Autodesk Inventor part; units mm, degrees
ref_plane "YZ Plane" through (0, 0, 0) normal (1, 0, 0) x (0, 1, 0)
ref_plane "XZ Plane" through (0, 0, 0) normal (0, 1, 0) x (-1, 0, 0)
ref_plane "XY Plane" through (0, 0, 0) normal (0, 0, 1) x (1, 0, 0)
sketch "Sketch2" plane through (0, 0, 0) normal (0, 0, 1) x (1, 0, 0)
  line L0 (-108, -20.3137) -> (62, -20.3137) construction
  line L1 (-108, -35.3137) -> (62, -35.3137)
  line L2 (62, -5.3137) -> (-108, -5.3137)
  arc A0 (-108, -5.3137) -> (-108, -35.3137) centre (-108, -20.3137) ccw
  arc A1 (62, -35.3137) -> (62, -5.3137) centre (62, -20.3137) ccw
  circle A2 centre (-108, -20.3137) radius 10
  circle A3 centre (62, -20.3137) radius 10
  line L3 (-84, -20.3137) -> (-68, -20.3137) construction
  line L4 (-84, -27.8137) -> (-68, -27.8137)
  line L5 (-68, -12.8137) -> (-84, -12.8137)
  arc A4 (-84, -12.8137) -> (-84, -27.8137) centre (-84, -20.3137) ccw
  arc A5 (-68, -27.8137) -> (-68, -12.8137) centre (-68, -20.3137) ccw
  line L6 (-23, -46) -> (-23, 6) construction
  arc A6 (-33, -27.8137) -> (-33, -12.8137) centre (-33, -20.3137) ccw
  line L7 (-49, -20.3137) -> (-33, -20.3137) construction
  line L8 (-49, -27.8137) -> (-33, -27.8137)
  line L9 (-33, -12.8137) -> (-49, -12.8137)
  arc A7 (-49, -12.8137) -> (-49, -27.8137) centre (-49, -20.3137) ccw
  line L10 (38, -20.3137) -> (22, -20.3137) construction
  line L11 (38, -27.8137) -> (22, -27.8137)
  line L12 (22, -12.8137) -> (38, -12.8137)
  arc A8 (38, -27.8137) -> (38, -12.8137) centre (38, -20.3137) ccw
  arc A9 (22, -12.8137) -> (22, -27.8137) centre (22, -20.3137) ccw
  arc A10 (-13, -12.8137) -> (-13, -27.8137) centre (-13, -20.3137) ccw
  line L13 (3, -20.3137) -> (-13, -20.3137) construction
  line L14 (3, -27.8137) -> (-13, -27.8137)
  line L15 (-13, -12.8137) -> (3, -12.8137)
  arc A11 (3, -27.8137) -> (3, -12.8137) centre (3, -20.3137) ccw
  line L16 (-121.6954, -14.1952) -> (-147.279, -14.1952)
  line L17 (-121.6954, -26.4323) -> (-147.279, -26.4323)
  circle A12 centre (-154, -20.3137) radius 9.0889
  circle A13 centre (-108, -20.3137) radius 12.5
  line L18 (-119.5282, -20.3137) -> (-121.5282, -20.3137)
  point P0 (0, 0)
  point P1 (-23, -20.3137)
  point P2 (-76, -20.3137)
  point P3 (-41, -20.3137)
  point P4 (30, -20.3137)
  point P5 (-5, -20.3137)
  point P6 (-120.5, -20.3137)
  dimension "d51" = 25
  dimension "d27" = 170
  dimension "d28" = 30
  dimension "d29" = 20
  dimension "d30" = 20
  dimension "d31" = 16
  dimension "d32" = 15
  dimension "d43" = 35
  dimension "d48" = 40
  dimension "d57" = 2
extrude "Extrusion2" add sketch "Sketch2" along normal blind 3 contours A0 L2 A1 L1 | L17 A12 L16 A0 | A12 | A13
extrude "Extrusion3" add sketch "Sketch2" against normal blind 3 contours A13
ref_plane "Work Plane1" through (-119.5282, -20.3137, 0) normal (0, -1, 0) x (-1, 0, 0)
sketch "Sketch4" plane through (-108, -20.3137, -3) normal (0, 0, -1) x (-1, 0, 0)
  line L0 (11.5282, 0) -> (13.5282, 0)
  circle A0 centre (0, 0) radius 12.5
  point P0 (-108, 20.3137)
  point P1 (12.5, 0)
ref_plane "Work Plane2" through (-120.5, -20.3137, -3) normal (-1, 0, 0) x (0, -1, 0)
sketch "Sketch5" plane through (-120.5, -20.3137, -3) normal (-1, 0, 0) x (0, -1, 0)
  line L0 (9.0889, 3) -> (-9.0889, 3)
  line L1 (-12.5, 0) -> (12.5, 0)
  line L2 (0, -1.2) -> (0, 7.2)
  line L3 (15, 3) -> (-15, 3)
  line L4 (0, 3) -> (0, 0)
  line L5 (10, 0) -> (-10, 0)
  line L6 (0, 3) -> (0, 0)
  circle A0 centre (0, 1.5) radius 0.25
  point P0 (-20.3137, 3)
  point P1 (-6.1186, 3)
  point P2 (6.1186, 3)
  dimension "d63" = 0.5
extrude "Extrusion5" cut sketch "Sketch5" against normal up to surface
pattern_circular "Circular Pattern1" count 3 over 360 about axis through (-108, -20.3137, 0) along (0, 0, -1) of "Extrusion5"
properties part number "p1"
Could you check a few things on this model? Use its own coordinates, in mm. A direction names the side the tool comes from. Round coordinates to 2 decimals unless told otherwise and drop trailing zeros. Write each loop counter-clockwise with the first axis right and the second up, starting at its lowest first coordinate (ties: lowest second). Pieces come first, ordered by that corner, then holes. Notation, with made-up numbers: M 14.5,-20 L 55.5,-20 A14 ccw 55.5,5 Z; hole C 81.5,7.25 d11. An arc over 180 degrees is marked long. Answer in a Markdown table with one row per item. Add a question column.
Q1. Imagine slicing it at B-B (z = 2). Please give me the cut outline in (x, y), then the cut area to 3 significant figures.
Q2. Will these pins go through, and if not, where does the flat tip stop? pin 1 Ø3 at (y, z) = (-23.5, -1) entering from +X; pin 2 Ø2.5 at (x, z) = (-129.5, 1) entering from -Y; pin 3 Ø1.5 at (x, z) = (-133, 1) entering from +Y.
Q3. If I drill on line 1 (Y direction, x = -108, z = -1.25); line 2 (Y direction, x = -108, z = 0.25); line 3 (Z direction, x = -89.5, y = -7.5), over which ranges is the centre line in solid material (lowest first)? Write a range as from..to.
Q4. On a 3-axis mill with a long thin cutter (end or side, diameter ignored), from which of +Z, -Z, +X, -X, +Y, -Y can I reach the whole of each face in a straight line? I mean faces 1 (the cylindrical face through (-96.077, -16.559, -1.479)), 2 (the cylindrical face through (-116, -33, 1)), 3 (the cylindrical face through (-20.5, -20.48, 1.48)). Say none if no direction works.
Q5. Imagine slicing it at C-C (x = -129.5). Please give me the cut outline in (y, z).
Q6. Imagine slicing it at A-A (x = -76.5). Please give me the cut outline in (y, z), then the cut area to 3 significant figures.
Values:
| question | item | result |
|---|---|---|
| 1 | outline | M -147.28,-26.43 L -121.7,-26.43 A15 ccw -108,-35.31 L 62,-35.31 A15 ccw 62,-5.31 L -108,-5.31 A15 ccw -121.7,-14.2 L -147.28,-14.2 A9.09 ccw long Z; hole C -108,-20.31 d20; hole M -84,-27.81 L -68,-27.81 A7.5 ccw -68,-12.81 L -84,-12.81 A7.5 ccw Z; hole M -49,-27.81 L -33,-27.81 A7.5 ccw -33,-12.81 L -49,-12.81 A7.5 ccw Z; hole M -13,-27.81 L 3,-27.81 A7.5 ccw 3,-12.81 L -13,-12.81 A7.5 ccw Z; hole M 22,-27.81 L 38,-27.81 A7.5 ccw 38,-12.81 L 22,-12.81 A7.5 ccw Z; hole C 62,-20.31 d20 |
| 1 | area | 4,050 mm^2 |
| 2 | pin 1 | x = 76.86 |
| 2 | pin 2 | y = -26.43 |
| 2 | pin 3 | y = -14.2 |
| 3 | line 1 | -32.81..-30.31, -10.31..-7.81 |
| 3 | line 2 | -35.31..-30.31, -10.31..-5.31 |
| 3 | line 3 | 0..3 |
| 4 | face 1 | -Z |
| 4 | face 2 | +Z, -Z, -Y |
| 4 | face 3 | +Z, -Z |
| 5 | outline | M -26.43,0 L -14.2,0 L -14.2,3 L -26.43,3 Z |
| 6 | outline | M -35.31,0 L -27.81,0 L -27.81,3 L -35.31,3 Z; M -12.81,0 L -5.31,0 L -5.31,3 L -12.81,3 Z |
| 6 | area | 45.0 mm^2 |
